Input: part model. Units: mm. Frame: model coordinates. Face numbers are marked on the shaded views. A direction names the side the tool comes from. Coordinates: 2 decimals unless noted, no trailing zeros. Write each loop counter-clockwise with the first axis right and the second up, starting at its lowest first coordinate (ties: lowest second). Pieces come first, ordered by that corner, then holes. Notation, with made-up numbers: (24.5, 78.25) -> (48.5, 78.25) arc R8 cw to (48.5, 89.25) -> close; hole circle Ø7 at (55, -2.75). An arc over 180 degrees is marked (long way). Use one line per item in the form item = value. Start each with the question number.
(1) Cut plane B-B on y = -4. Return the cut outline in (x, z), plus the area to 3 significant figures.
(2) Cut plane A-A on y = -0.75. Return the cut outline in (x, z), plus the area to 3 significant figures.
(3) First-contact query: pin 1 (2.5 mm diameter, centred on x = 15.5, y = -0.5, fed in from -Z); pin 2 (1.5 mm diameter, centred on x = 16, y = 1, fed in from +Z); pin 3 (10 mm diameter, centred on x = 24.5, z = 9, fed in from +Y); pin 4 (1.5 mm diameter, centred on y = 3.5, z = -12.5, fed in from +X). Flat tips, straight axial feed; report the tip coordinate or a pass-through.
(4) Ray query, line 1 along X through (y, z) = (-3.7, 0); line 2 along X through (y, z) = (-0.9, -30); line 3 along X through (y, z) = (-3.5, 28). Return the intervals inside material, ascending.
(5) Cut plane C-C on x = 4.5. Return the cut outline in (y, z).
(6) Pull-direction query (Z, two-part tool) for the marked faces 1, 2 and 3; classes: released by +Z, released by -Z, zero draft, split by the parting line, or undercut.
(7) Cut plane D-D on x = 0. Return the cut outline in (y, z), plus the area to 3 significant figures.
(8) Set-up query: the marked faces 4 and 5. Return all of +Z, -Z, +X, -X, +Y, -Y with unobstructed straight access to the full face (end or side cutting, diameter ignored); none if empty.
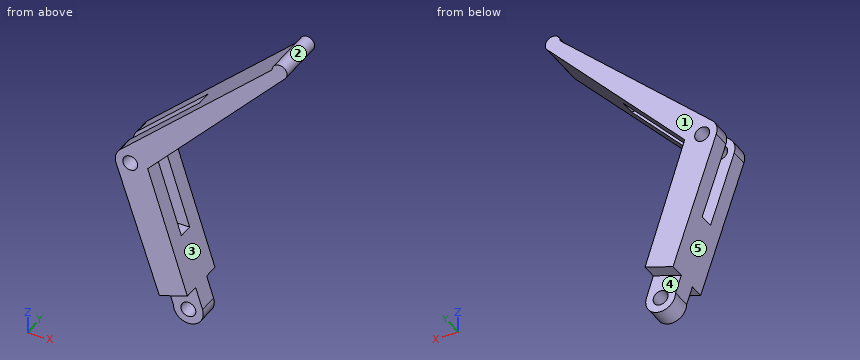
```python
from build123d import *

# Parameters (mm, degrees)
CROQUIS1_R                 = 1.5
SALIENTE_EXTRUIR1_DEPTH    = 5
CORTAR_EXTRUIR1_DEPTH      = 45.551969752
CORTAR_EXTRUIR1_DEPTH_BACK = 45.551969752
CROQUIS2_W                 = 7.521993914
CROQUIS2_H                 = 3
CORTAR_EXTRUIR2_DEPTH      = 46.893899377
CORTAR_EXTRUIR2_DEPTH_BACK = 46.893899377
CROQUIS3_W                 = 30
CROQUIS3_H                 = 3


with BuildPart() as part:
    # Croquis1 → Saliente-Extruir1 (new, symmetric)
    with BuildSketch(Plane(origin=(0, 0, 0), x_dir=(1, 0, 0), z_dir=(0, 1, 0))):
        with BuildLine():
            Line((28.5, -30), (-2.01947172, -2.218498134))
            ThreePointArc((-2.01947172, -2.218498134), (-2.904664292, -0.750283514), (-2.84125158, 0.962958702))
            Line((-2.84125158, 0.962958702), (7, 30))
            ThreePointArc((7, 30), (10.465003416, 32.963742874), (12.855847882, 29.081232959))
            Line((12.855847882, 29.081232959), (3.5, 0))
            Line((3.5, 0), (31.086206897, -28.965517241))
            ThreePointArc((31.086206897, -28.965517241), (30.557086015, -31.392715036), (28.5, -30))
        make_face()
        with Locations(Location((10, 30, 0), (0, 0, 270))):
            Circle(CROQUIS1_R, mode=Mode.SUBTRACT)
        with Locations(Location((0, 0, 0), (0, 0, 270))):
            Circle(CROQUIS1_R, mode=Mode.SUBTRACT)
    extrude(amount=SALIENTE_EXTRUIR1_DEPTH, both=True)

    # Croquis2 → Cortar-Extruir1 (cut, two sides: drawn at the far end of the back side and taken through both)
    with BuildSketch(Plane(origin=(3.171726104, 0, 1.020389575), x_dir=(0.3062556803556079, 0, -0.9519492939489601), z_dir=(0.9519492939489601, 0, 0.3062556803556079)).offset(-CORTAR_EXTRUIR1_DEPTH_BACK)):
        with Locations((30.860038665, -3.5)):
            Rectangle(CROQUIS2_W, CROQUIS2_H)
        with Locations((30.860038665, 3.5)):
            Rectangle(CROQUIS2_W, CROQUIS2_H)
    extrude(amount=CORTAR_EXTRUIR1_DEPTH + CORTAR_EXTRUIR1_DEPTH_BACK, mode=Mode.SUBTRACT)

    # Croquis3 → Cortar-Extruir2 (cut, two sides: drawn at the far end of the back side and taken through both)
    with BuildSketch(Plane(origin=(0, 0, 0), x_dir=(0, 0, -1), z_dir=(1, 0, 0)).offset(-CORTAR_EXTRUIR2_DEPTH_BACK)):
        Rectangle(CROQUIS3_W, CROQUIS3_H)
    extrude(amount=CORTAR_EXTRUIR2_DEPTH + CORTAR_EXTRUIR2_DEPTH_BACK, mode=Mode.SUBTRACT)


solid = part.part
```
Values:
q1.outline = (-2.84, -0.96) -> (5.84, -26.59) -> (11.47, -24.78) -> (3.5, 0) -> (31.09, 28.97) arc R1.5 ccw (long way) to (28.5, 30) -> (-2.02, 2.22) arc R3 ccw to start; hole circle Ø3 at (0, 0)
q1.area = 333 mm2
q2.outline = (1.92, -15) -> (7, -30) arc R3 ccw (long way) to (12.86, -29.08) -> (8.33, -15) -> close; (12.02, 15) -> (17.79, 15) -> (31.09, 28.97) arc R1.5 ccw (long way) to (28.5, 30) -> close; hole circle Ø3 at (10, -30)
q2.area = 175 mm2
q3.pin_1 = 11.81
q3.pin_2 = 19.3
q3.pin_3 = through
q3.pin_4 = 7.76
q4.line_1 = -3 to -1.5, 1.5 to 3.5
q4.line_2 = 7 to 8.5, 11.5 to 13
q4.line_3 = 26.3 to 30.17
q5.outline = (-5, -22.62) -> (5, -22.62) -> (5, -3.11) -> (1.5, -3.11) -> (1.5, -15) -> (-1.5, -15) -> (-1.5, -3.11) -> (-5, -3.11) -> close; (-5, 1.05) -> (-1.5, 1.05) -> (-1.5, 8.15) -> (-5, 8.15) -> close; (1.5, 1.05) -> (5, 1.05) -> (5, 8.15) -> (1.5, 8.15) -> close
q6.face_1 = zero draft
q6.face_2 = split by the parting line
q6.face_3 = undercut
q7.outline = (-5, -9.35) -> (-1.5, -9.35) -> (-1.5, -1.5) -> (-5, -1.5) -> close; (-5, 1.5) -> (-1.5, 1.5) -> (-1.5, 4.06) -> (-5, 4.06) -> close; (1.5, -9.35) -> (5, -9.35) -> (5, -1.5) -> (1.5, -1.5) -> close; (1.5, 1.5) -> (5, 1.5) -> (5, 4.06) -> (1.5, 4.06) -> close
q7.area = 72.8 mm2
q8.face_4 = -Z, +X, +Y
q8.face_5 = -Z, -X, +Y, -Y
